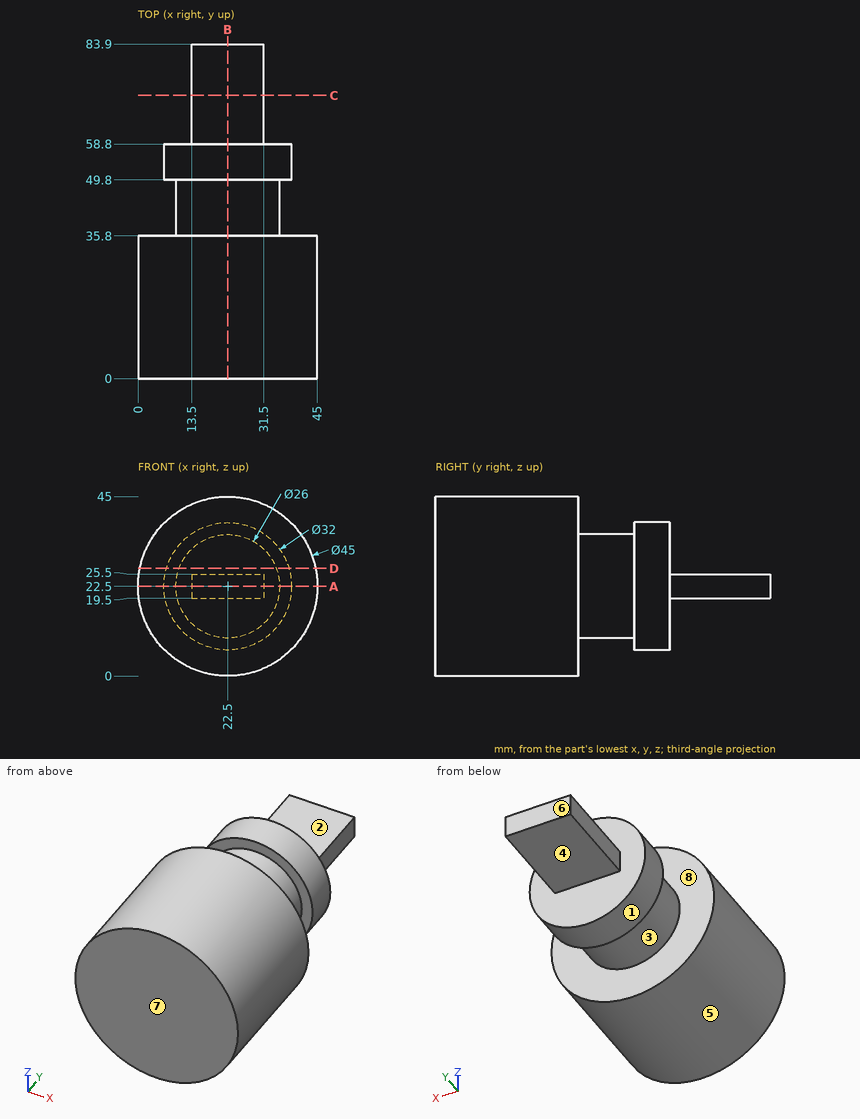
For this review, use the dimensioned drawing (mm, ordinates from the lowest corner) and the shaded views. A direction names the side the tool comes from. Coordinates: 2 decimals unless noted, no trailing zeros. Write each loop counter-clockwise with the first axis right and the second up, starting at its lowest first coordinate (ties: lowest second). Pieces come first, ordered by that corner, then holes. Notation, with made-up numbers: (-39.5, 70) - (-18.5, 70) arc R36 cw to (-18.5, 105) - close; hole circle Ø1 at (15, 4). An arc over 180 degrees is marked (long way). Answer in a Markdown table with one row per item. Add a question column.
Q1. Consider section D-D on z = 27. Give the boundary of the cut face in (x, y).
Q2. Consider section C-C on y = 71. Give the boundary of the cut face in (x, z), then the cut area to 3 significant figures.
Q3. Consider section A-A on z = 22.5. Give the boundary of the cut face in (x, y).
Q4. Consider section B-B on x = 22.5. Give the boundary of the cut face in (y, z).
Q5. To check wall thickness, follow line 1 along Y through (x, z) = (30.5, 10); line 2 along Y through (x, z) = (20, 32); line 3 along Y through (x, z) = (23, 41.5). State the ranges of each line that lie inside material, in increasing order. Write a range as from..to.
Q6. For the marked faces 1, 2, 3 and 4, list the 3-axis set-ups (+Z, -Z, +X, -X, +Y, -Y) from which the entire face can be reached by the end or side of a thin tool; tool diameter is ignored.
Q7. Draft analysis for pull direction Y (two halves, no side actions). For the marked faces 5, 6, 7 and 8, state which applies: +Y half, -Y half, draft (parallel to the pull), parting line (faces both ways), or undercut.
Q8. Clearance check with flat-ended pins moving along their axes: pin 1 (8 mm diameter, centred on x = 28.5, y = 22, fed in from -Z); pin 2 (1.5 mm diameter, centred on x = 15.5, z = 35.5, fed in from +Y); pin 3 (10 mm diameter, centred on x = 19, y = 37.5, fed in from +Z). State where each tip first meets the part, or that it passes through.
Answers below:
| question | item | result |
|---|---|---|
| 1 | outline | (0.45, 0) - (44.55, 0) - (44.55, 35.8) - (34.7, 35.8) - (34.7, 49.8) - (37.85, 49.8) - (37.85, 58.8) - (7.15, 58.8) - (7.15, 49.8) - (10.3, 49.8) - (10.3, 35.8) - (0.45, 35.8) - close |
| 2 | outline | (13.5, 19.5) - (31.5, 19.5) - (31.5, 25.5) - (13.5, 25.5) - close |
| 2 | area | 108 mm² |
| 3 | outline | (0, 0) - (45, 0) - (45, 35.8) - (35.5, 35.8) - (35.5, 49.8) - (38.5, 49.8) - (38.5, 58.8) - (31.5, 58.8) - (31.5, 83.9) - (13.5, 83.9) - (13.5, 58.8) - (6.5, 58.8) - (6.5, 49.8) - (9.5, 49.8) - (9.5, 35.8) - (0, 35.8) - close |
| 4 | outline | (0, 0) - (35.8, 0) - (35.8, 9.5) - (49.8, 9.5) - (49.8, 6.5) - (58.8, 6.5) - (58.8, 19.5) - (83.9, 19.5) - (83.9, 25.5) - (58.8, 25.5) - (58.8, 38.5) - (49.8, 38.5) - (49.8, 35.5) - (35.8, 35.5) - (35.8, 45) - (0, 45) - close |
| 5 | line 1 | 0..35.8, 49.8..58.8 |
| 5 | line 2 | 0..58.8 |
| 5 | line 3 | 0..35.8 |
| 6 | face 1 | +Y |
| 6 | face 2 | +Z, +X, -X, +Y |
| 6 | face 3 | none |
| 6 | face 4 | -Z, +X, -X, +Y |
| 7 | face 5 | draft |
| 7 | face 6 | +Y half |
| 7 | face 7 | -Y half |
| 7 | face 8 | undercut |
| 8 | pin 1 | z = 0.09 |
| 8 | pin 2 | y = 58.8 |
| 8 | pin 3 | z = 45 |
